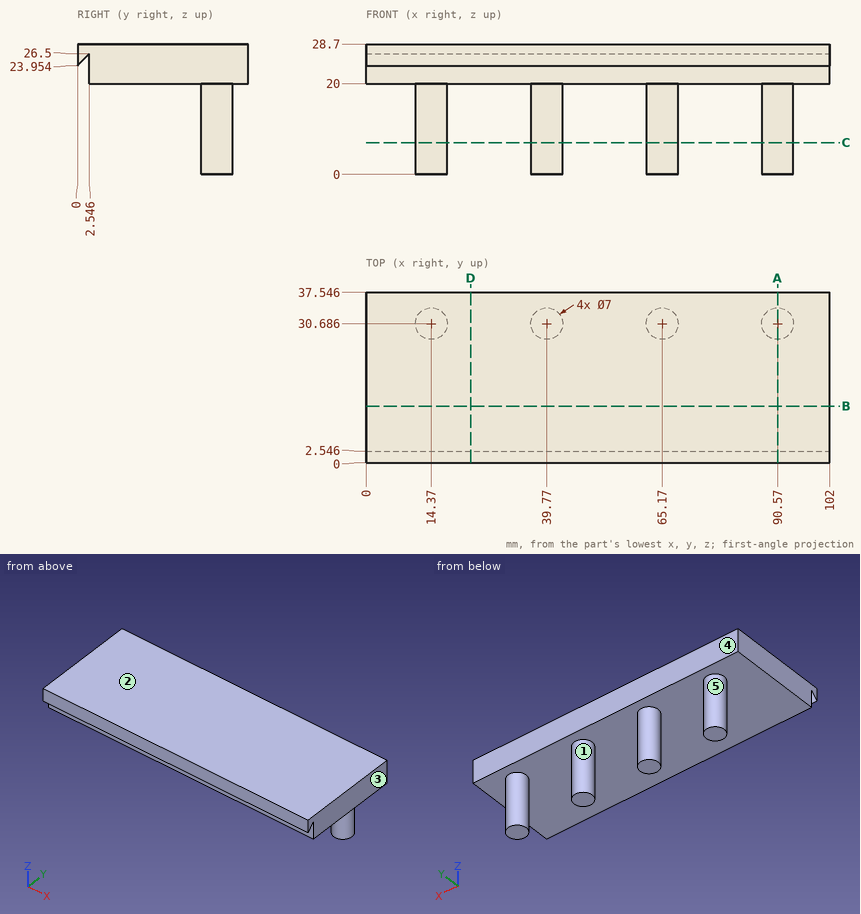
Geometry check sheet. Reference: drawing and pictorial views, mm from the part's lowest x, y, z. A direction names the side the tool comes from. Give positions to 0.01 mm unless a question says otherwise; leave off trailing zeros. Loops run counter-clockwise (first coordinate to the right, second up) from the corner with the lowest first, then second, coordinate; pieces in that order, holes last. Notation, with made-up numbers: (48.25, 78.5) -> (76.25, 78.5) arc R35 cw to (76.25, 115.5) -> close; hole circle Ø9 at (84, 24.5). An arc over 180 degrees is marked (long way). Answer in a Markdown table with one row per item. Add a question column.
1) Cross-section at D-D on x = 23. Record the boundary of the cut face in (y, z) (1 decimal).
2) Gauge pin test, flat ends, axial feed: P1, Ø1, axis at y = 28.5, z = 10.5, coming from the -X side; P2, Ø4, axis at x = 50.5, y = 18, coming from the -Z side; P3, Ø2, axis at x = 29, z = 22, coming from the -Y side. Record the tip position at first contact, or that the pin passes through.
3) Draft check along X on the marked faces 1, 2 and 3. Enter one of: pulls with the +X half, pulls with the -X half, needs draft (parallel to the pull), parting line crosses it, or undercut.
4) Cross-section at A-A on x = 90.57. Record the boundary of the cut face in (y, z) (1 decimal).
5) Cross-section at C-C on z = 7. Record the boundary of the cut face in (x, y) (1 decimal).
6) Material ranges on probe 1 along Y at (x, z) = (46, 23) (1 decimal); probe 2 along Z at (x, y) = (89.5, 8.5); probe 3 along Y at (x, z) = (39.5, 25.5) (1 decimal), recorded low to high. Write a range as from..to.
7) Cross-section at B-B on y = 12.5. Record the boundary of the cut face in (x, z).
8) Set-up check for the marked faces 4 and 5: record each of +Z, -Z, +X, -X, +Y, -Y from which the full face is reachable in a straight line by a thin tool's end or side.
Outcome:
| question | item | result |
|---|---|---|
| 1 | outline | (0, 24) -> (2.5, 26.5) -> (2.5, 20) -> (37.5, 20) -> (37.5, 28.7) -> (0, 28.7) -> close |
| 2 | P1 | stops at x = 11.3 |
| 2 | P2 | stops at z = 20 |
| 2 | P3 | stops at y = 2.55 |
| 3 | face 1 | undercut |
| 3 | face 2 | needs draft |
| 3 | face 3 | pulls with the +X half |
| 4 | outline | (0, 24) -> (2.5, 26.5) -> (2.5, 20) -> (27.2, 20) -> (27.2, 0) -> (34.2, 0) -> (34.2, 20) -> (37.5, 20) -> (37.5, 28.7) -> (0, 28.7) -> close |
| 5 | outline | circle Ø7 at (14.4, 30.7); circle Ø7 at (39.8, 30.7); circle Ø7 at (65.2, 30.7); circle Ø7 at (90.6, 30.7) |
| 6 | probe 1 | y = 2.5..37.5 |
| 6 | probe 2 | z = 20..28.7 |
| 6 | probe 3 | y = 0..1.5, 2.5..37.5 |
| 7 | outline | (0, 20) -> (102, 20) -> (102, 28.7) -> (0, 28.7) -> close |
| 8 | face 4 | +Z, -Z, +X, -X, +Y |
| 8 | face 5 | -Z |
